The drawing under review shows one solid part. Ordinate dimensions are in mm from its lowest x, y, z. A direction names the side the tool comes from. Give positions to 0.01 mm unless a question says otherwise; leave off trailing zeros. Loops run counter-clockwise (first coordinate to the right, second up) from the corner with the lowest first, then second, coordinate; pieces in that order, holes last. Notation, with made-up numbers: M 44.5,-17 L 83.5,-17 A19 cw 83.5,3 Z; hole C -28,-1.75 d6. An arc over 180 degrees is marked long. Put each result on its own line as item: value. Start each with the question number.
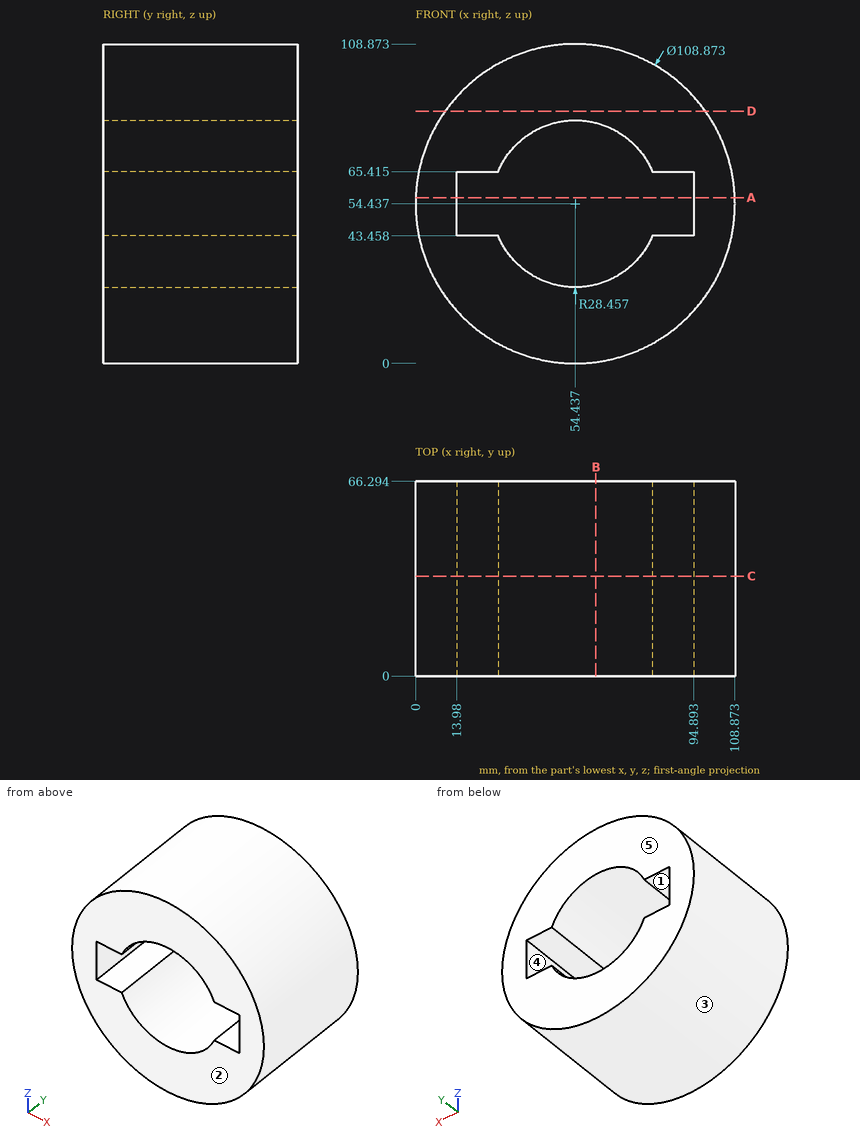
Item 1: Clearance check with flat-ended pins moving along their axes: pin 1 Ø4 at (x, y) = (58.5, 9.5) entering from -Z; pin 2 Ø1 at (x, y) = (43.5, 14.5) entering from -Z; pin 3 Ø1 at (y, z) = (45.5, 66) entering from +X. State where each tip first meets the part, or that it passes through.
Item 2: To check wall thickness, follow L1, parallel to Z at x = 44, y = 48.5; L2, parallel to X at y = 56, z = 75.5 (1 decimal); L3, parallel to Z at x = 81.5, y = 39.5 (1 decimal). State the ranges of each line that lie inside material, in increasing order. Write a range as [from, to].
Item 3: Consider section C-C, the plane y = 34. Write out the cut boundary in (x, z) (1 decimal), plus the area to 3 significant figures.
Item 4: Consider section D-D, the plane z = 86. Write out the cut boundary in (x, y) (1 decimal).
Item 5: Consider section A-A, the plane z = 56.5. Write out the cut boundary in (x, y).
Item 6: Draft analysis for pull direction Z (two halves, no side actions). For the marked faces 3, 4 and 5, state which applies: +Z half, -Z half, draft (parallel to the pull), parting line (faces both ways), or undercut.
Item 7: Tool access review of the marked faces 1 and 2: name each direction out of +Z, -Z, +X, -X, +Y, -Y from which nothing blocks a thin tool from reaching the whole face with its end or side.
Item 8: Consider section B-B, the plane x = 61.5. Write out the cut boundary in (y, z).
Report:
1. pin 1: z = 0.04
1. pin 2: z = 1.01
1. pin 3: x = 107.74
2. L1: [1.01, 27.96], [80.91, 107.86]
2. L2: [4.2, 35.3], [73.6, 104.6]
2. L3: [7.2, 43.5], [65.4, 101.7]
3. outline: C 54.4,54.4 d108.9; hole M 14,43.5 L 28.2,43.5 A28.5 ccw 80.7,43.5 L 94.9,43.5 L 94.9,65.4 L 80.7,65.4 A28.5 ccw 28.2,65.4 L 14,65.4 Z
3. area: 6,210 mm²
4. outline: M 10.1,0 L 98.8,0 L 98.8,66.3 L 10.1,66.3 Z
5. outline: M 0.04,0 L 13.98,0 L 13.98,66.29 L 0.04,66.29 Z; M 94.89,0 L 108.83,0 L 108.83,66.29 L 94.89,66.29 Z
6. face 3: parting line
6. face 4: undercut
6. face 5: draft
7. face 1: +Y, -Y
7. face 2: +Z, -Z, +X, -X, -Y
8. outline: M 0,0.46 L 66.29,0.46 L 66.29,26.87 L 0,26.87 Z; M 0,82 L 66.29,82 L 66.29,108.41 L 0,108.41 Z
